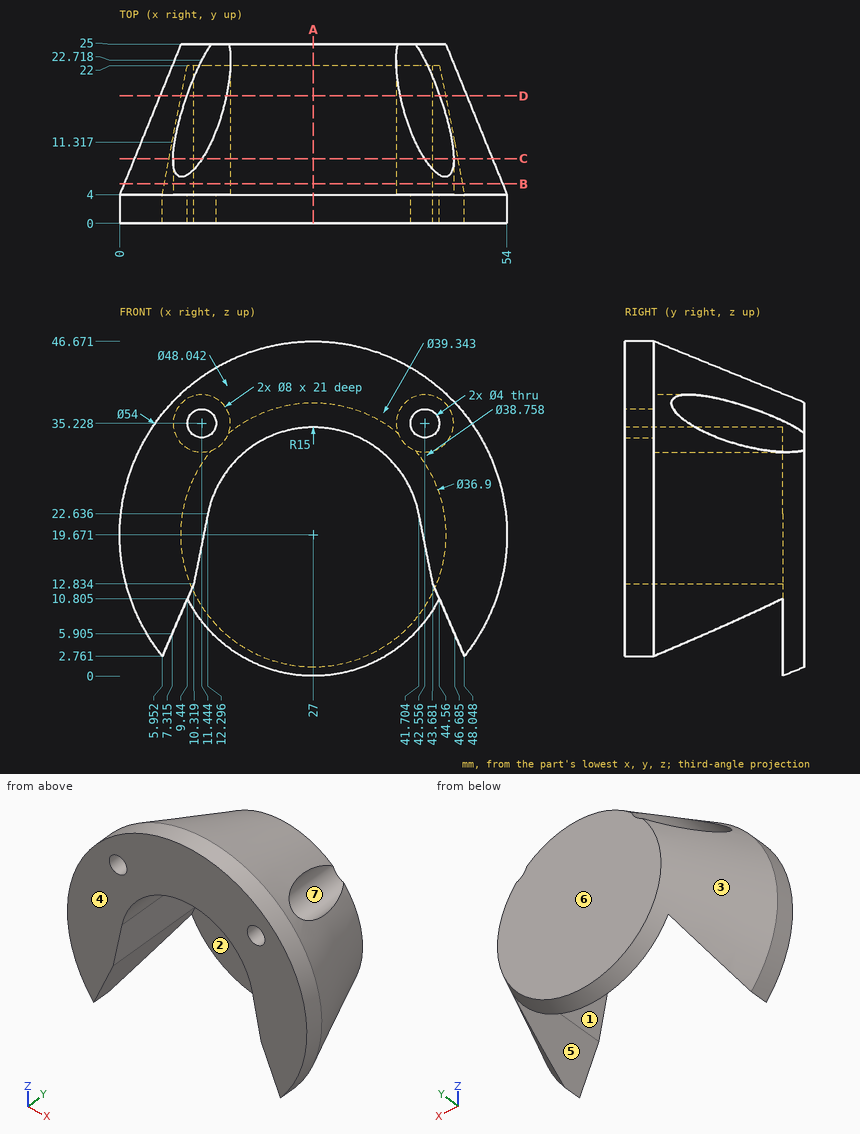
Can you work these out from the drawing? Everything is in mm from the part's minimum corner. A direction names the side the tool comes from. Round coordinates to 2 decimals unless told otherwise and drop trailing zeros. Order: outer loops, then holes, each group sorted by start corner. A loop starts at its lowest first (then second) coordinate and runs counter-clockwise, first axis right, second up. Notation, with made-up numbers: M -32.5,-17.75 L 4.5,-17.75 A25 ccw 4.5,2.25 Z; hole C -25.75,-39.75 d8. An arc over 180 degrees is marked long. Answer as CSV lines item,"result".
Item 1: We'd pull the mould along X, two halves only. Please class the marked faces 1, 2, 3 and 4: +X half, -X half, draft (parallel to the pull), parting line (faces both ways), or undercut.
From the geometry:
face 1,"undercut"
face 2,"undercut"
face 3,"parting line"
face 4,"draft"
Item 2: Please list where these lines run through material, in increasing order: L1, parallel to Y at x = 41, z = 10; L2, parallel to X at y = 3.25, z = 8.5; L3, parallel to X at y = 22.25, z = 19. Write a range as [from, to].
From the geometry:
L1,"[22, 25]"
L2,"[2.42, 8.44], [45.56, 51.58]"
L3,"[7.44, 46.56]"
Item 3: Imagine slicing it at A-A on x = 27. List the corners of the cut face in (y, z) for me.
From the geometry:
outline,"M 0,34.67 L 22,34.67 L 22,0 L 25,1.22 L 25,38.12 L 4,46.67 L 0,46.67 Z"
Item 4: Which directions (+Z, -Z, +X, -X, +Y, -Y) give clear straight access to the entire face, cutting with the end or side of a thin tool? Please do the marked faces 5, 6 and 7.
From the geometry:
face 5,"-Z, -Y"
face 6,"+Z, -Z, +X, -X, +Y"
face 7,"+Y"
Item 5: Imagine slicing it at B-B on y = 5.5. List the corners of the cut face in (x, z) for me (1 decimal).
From the geometry:
outline,"M 6.2,3.4 L 10.3,12.8 L 12.3,22.6 A15 cw 41.7,22.6 L 43.7,12.8 L 47.8,3.4 A26.4 ccw long Z; hole C 11.4,35.2 d8; hole C 42.6,35.2 d8"
Item 6: For pin 1 (1.5 mm diameter, centred on y = 22, z = 33, fed in from +X) (1 decimal); pin 2 (8 mm diameter, centred on y = 3, z = 10, fed in from +X); pin 3 (2.5 mm diameter, centred on x = 42.56, z = 35.23, fed in from -Y); pin 4 (6.5 mm diameter, centred on x = 42.56, z = 35.23, fed in from +Y), each with a flat end and sliding along its axis, tell me the tip position at first contact or that it passes through.
From the geometry:
pin 1,"x = 39.9"
pin 2,"x = 53.4"
pin 3,"through"
pin 4,"y = 4"
Item 7: Imagine slicing it at D-D on y = 17.75. List the corners of the cut face in (x, z) for me (1 decimal).
From the geometry:
outline,"M 8.6,8.8 L 10.3,12.8 L 12.3,22.6 A15 cw 41.7,22.6 L 43.7,12.8 L 45.4,8.8 A21.4 ccw 44.6,31.8 A4 cw 39.1,37.3 A21.4 ccw 14.9,37.3 A4 cw 9.4,31.8 A21.4 ccw Z"
Item 8: Imagine slicing it at C-C on y = 9. List the corners of the cut face in (x, z) for me (1 decimal), and give its area (3 significant figures).
From the geometry:
outline,"M 6.9,4.9 L 10.3,12.8 L 12.3,22.6 A15 cw 41.7,22.6 L 43.7,12.8 L 47.1,4.9 A25 ccw 46.6,35.2 A4 cw long 42.5,39.2 A25 ccw 11.5,39.2 A4 cw long 7.4,35.2 A25 ccw Z"
area,"714 mm2"
